Can you work these out from the drawing? Everything is in mm from the part's minimum corner. Round coordinates to 2 decimals unless told otherwise and drop trailing zeros. Write each loop counter-clockwise with the first axis right and the second up, starting at its lowest first coordinate (ties: lowest second). Pieces come first, ordered by that corner, then holes. Notation, with made-up numbers: (89.5, 21) - (127.5, 21) arc R19 ccw to (127.5, 41) - close; hole circle Ø7 at (34, 3.5). An arc over 180 degrees is marked (long way). One line per item, written item: value. Start each with the question number.
Item 1: For P1, Ø5, axis at x = 24, z = 65.05, coming from the +Y side; P2, Ø1, axis at x = 38, y = 0.5, coming from the +Z side, each with a flat end and sliding along its axis, tell me the tip position at first contact or that it passes through.
Item 2: Imagine slicing it at C-C, the plane x = 56. Please give me the cut outline in (y, z) (3 decimals), then the cut area to 3 significant figures.
Item 3: Imagine slicing it at D-D, the plane y = 0.35. Count the separate pieces of the cut face and the enclosed holes in it, then the cut area to 3 significant figures.
Item 4: Imagine slicing it at A-A, the plane x = 31. Please give me the cut outline in (y, z).
Item 5: Imagine slicing it at B-B, the plane z = 89.05. Please give me the cut outline in (x, y) (3 decimals).
Item 6: If I drill on line 1 (X direction, y = 1.55, z = 65.05) (3 decimals); line 2 (X direction, y = 1, z = 5.05) (3 decimals); line 3 (Z direction, x = 55, y = 0.3), over which ranges is the centre line in solid material (lowest first)?
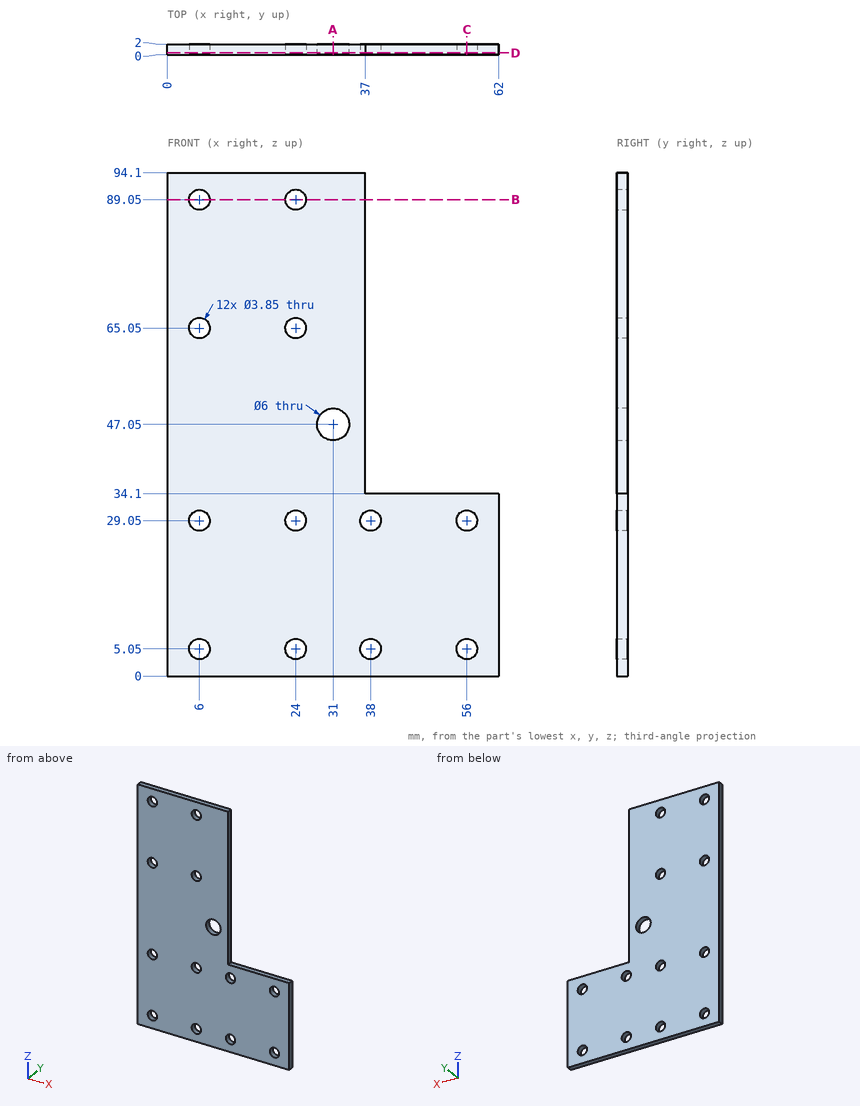
Values follow:
1. P1: stops at y = 2
1. P2: stops at z = 34.1
2. outline: (0, 0) - (2, 0) - (2, 3.125) - (0, 3.125) - close; (0, 6.975) - (2, 6.975) - (2, 27.125) - (0, 27.125) - close; (0, 30.975) - (2, 30.975) - (2, 34.1) - (0, 34.1) - close
2. area: 52.8 mm^2
3. separate pieces: 1
3. enclosed holes: 13
3. area: 4,170 mm^2
4. outline: (0, 0) - (2, 0) - (2, 44.05) - (0, 44.05) - close; (0, 50.05) - (2, 50.05) - (2, 94.1) - (0, 94.1) - close
5. outline: (0, 0) - (4.075, 0) - (4.075, 2) - (0, 2) - close; (7.925, 0) - (22.075, 0) - (22.075, 2) - (7.925, 2) - close; (25.925, 0) - (37, 0) - (37, 2) - (25.925, 2) - close
6. line 1: x = 0 to 4.075, 7.925 to 22.075, 25.925 to 37
6. line 2: x = 0 to 4.075, 7.925 to 22.075, 25.925 to 36.075, 39.925 to 54.075, 57.925 to 62
6. line 3: z = 0 to 3.41, 6.69 to 27.41, 30.69 to 34.1
